from build123d import *

# Parameters (mm, degrees)
SKETCH1_W           = 60
SKETCH1_H           = 80
BOSS_EXTRUDE1_DEPTH = 10
SKETCH3_W           = 45
SKETCH3_H           = 40
CUT_EXTRUDE1_DEPTH  = 51.990195136
SKETCH4_W           = 45
SKETCH4_H           = 20
CUT_EXTRUDE2_DEPTH  = 51.990195136
SKETCH5_R           = 2
CUT_EXTRUDE3_DEPTH  = 73.801098893
FILLET1_R           = 5
SKETCH6_W           = 36
SKETCH6_H           = 25
CUT_EXTRUDE4_DEPTH  = 51.990195136


with BuildPart() as part:
    # Sketch1 → Boss-Extrude1 (new body)
    with BuildSketch(Plane(origin=(0, 0, 0), x_dir=(1, 0, 0), z_dir=(0, 1, 0))):
        Rectangle(SKETCH1_W, SKETCH1_H)
    extrude(amount=BOSS_EXTRUDE1_DEPTH)

    # Sketch3 → Cut-Extrude1 (cut, through all)
    with BuildSketch(Plane(origin=(0, 10, 0), x_dir=(1, 0, 0), z_dir=(0, 1, 0))):
        with Locations((0, 20)):
            Rectangle(SKETCH3_W, SKETCH3_H)
    extrude(amount=-CUT_EXTRUDE1_DEPTH, mode=Mode.SUBTRACT)

    # Sketch4 → Cut-Extrude2 (cut, through all)
    with BuildSketch(Plane(origin=(0, 10, 0), x_dir=(1, 0, 0), z_dir=(0, 1, 0))):
        with Locations((0, -30)):
            Rectangle(SKETCH4_W, SKETCH4_H)
    extrude(amount=-CUT_EXTRUDE2_DEPTH, mode=Mode.SUBTRACT)

    # Sketch5 → Cut-Extrude3 (cut, through all)
    with BuildSketch(Plane.ZY.offset(30)):
        with Locations((35, 5)):
            Circle(SKETCH5_R)
        with Locations((-35, 5)):
            Circle(SKETCH5_R)
    extrude(amount=-CUT_EXTRUDE3_DEPTH, mode=Mode.SUBTRACT)

    # Fillet1
    fillet1_edges = [part.edges().sort_by_distance(p)[0] for p in [
        (26.25, 0, 40),
        (-26.25, 0, 40),
        (-26.25, 0, -40),
        (26.25, 0, -40),
        (-26.25, 10, -40),
        (-26.25, 10, 40),
        (26.25, 10, 40),
        (26.25, 10, -40),
    ]]
    fillet(fillet1_edges, radius=FILLET1_R - 0.0001)  # a hair under: the kernel refuses the full size

    # Sketch6 → Cut-Extrude4 (cut, through all)
    with BuildSketch(Plane(origin=(0, 10, 0), x_dir=(1, 0, 0), z_dir=(0, 1, 0))):
        Rectangle(SKETCH6_W, SKETCH6_H)
    extrude(amount=-CUT_EXTRUDE4_DEPTH, mode=Mode.SUBTRACT)


solid = part.part
The model under review builds one solid part; all positions refer to its coordinate system, in mm. A direction names the side the tool comes from. Give positions to 0.01 mm unless a question says otherwise; leave off trailing zeros. Loops run counter-clockwise (first coordinate to the right, second up) from the corner with the lowest first, then second, coordinate; pieces in that order, holes last. Notation, with made-up numbers: (78, 33) -> (91, 33) arc R22 ccw to (91, 55) -> close; hole circle Ø5 at (26, 36). An arc over 180 degrees is marked (long way). Put each result on its own line as item: value. Start each with the question number.
1. We need section D-D on y = 9. State the section outline as (x, z) points, then the cut area to 3 significant figures.
2. We need section C-C on z = 9. State the section outline as (x, y) points, then the cut area to 3 significant figures.
3. We need section A-A on z = -29. State the section outline as (x, y) points, then the cut area to 3 significant figures.
4. For faces 5 (the face through (-22.5, 5, 30)), 6 (the face through (20, 5, 0)), 7 (the face through (0, 10, 13)), list the 3-axis set-ups (+Z, -Z, +X, -X, +Y, -Y) from which the entire face can be reached by the end or side of a thin tool; tool diameter is ignored.
5. Wall thickness on probe 1 along X at (y, z) = (1.25, -20); probe 2 along X at (y, z) = (8.5, 2); probe 3 along Z at (x, y) = (24, 5.75): over which ranges is each line inside the solid? List them lowest first.
6. Mouldability with a two-part tool opening along X and no side actions: class faces 1 (the face through (-18, 5, 6)), 2 (the face through (-30, 5, 1)), 3 (the face through (-22.5, 5, -20)), 4 (the face through (-26.303, 5.601, -33.092)) as released by +X, released by -X, zero draft, split by the parting line, or undercut.
7. We need section B-B on x = 23.5. State how many separate pieces and enclosed holes the cut face has, then the cut area to 3 significant figures.
8. Clearance check with flat-ended pins moving along their axes: P1, Ø6, axis at x = -11, y = 8.5, coming from the -Z side; P2, Ø5, axis at x = 21, y = 3, coming from the -Z side; P3, Ø8, axis at x = 16.5, z = -11, coming from the +Y side; P4, Ø3, axis at x = 9, y = 5, coming from the +Z side. State where each tip first meets the part, or that it passes through.
Determined:
1. outline: (-30, -38) -> (-22.5, -38) -> (-22.5, 0) -> (-18, 0) -> (-18, 12.5) -> (18, 12.5) -> (18, 0) -> (22.5, 0) -> (22.5, -38) -> (30, -38) -> (30, 38) -> (22.5, 38) -> (22.5, 20) -> (-22.5, 20) -> (-22.5, 38) -> (-30, 38) -> close
1. area: 1,590 mm^2
2. outline: (-30, 0) -> (-18, 0) -> (-18, 10) -> (-30, 10) -> close; (18, 0) -> (30, 0) -> (30, 10) -> (18, 10) -> close
2. area: 240 mm^2
3. outline: (-30, 0) -> (-22.5, 0) -> (-22.5, 10) -> (-30, 10) -> close; (22.5, 0) -> (30, 0) -> (30, 10) -> (22.5, 10) -> close
3. area: 150 mm^2
4. face 5: +Z, +Y, -Y
4. face 6: -Z, +Y, -Y
4. face 7: +Z, -Z, +X, -X, +Y
5. probe 1: -30 to -22.5, 22.5 to 30
5. probe 2: -30 to -18, 18 to 30
5. probe 3: -39.94 to -36.85, -33.15 to 33.15, 36.85 to 39.94
6. face 1: undercut
6. face 2: released by -X
6. face 3: undercut
6. face 4: zero draft
7. separate pieces: 1
7. enclosed holes: 2
7. area: 753 mm^2
8. P1: z = 12.5
8. P2: z = -40
8. P3: through
8. P4: z = 20
